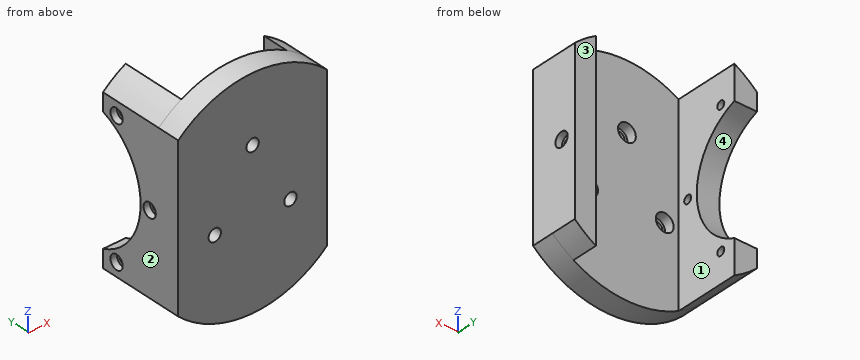
```python
from build123d import *

# Parameters (mm, degrees)
SKETCH8_R            = 1.912019499
BOSS_EXTRUDE7_DEPTH  = 7
SKETCH9_R            = 2.75
CUT_EXTRUDE4_DEPTH   = 3
BOSS_EXTRUDE9_DEPTH  = 20
SKETCH13_R           = 20.5
CUT_EXTRUDE7_DEPTH   = 19.5
SKETCH14_R           = 1.25
CUT_EXTRUDE8_DEPTH   = 19.5
SKETCH15_R           = 2.2
CUT_EXTRUDE9_DEPTH   = 2
BOSS_EXTRUDE10_DEPTH = 8
SKETCH17_R           = 1.25
CUT_EXTRUDE10_DEPTH  = 7.5
CUT_EXTRUDE11_START  = -2
SKETCH18_R           = 2.2
CUT_EXTRUDE11_DEPTH  = 2


with BuildPart() as part:
    # Sketch8 → Boss-Extrude7 (new body)
    with BuildSketch(Plane(origin=(0, 0, 0), x_dir=(1, 0, 0), z_dir=(0, 1, 0))):
        with BuildLine():
            Line((-23, 24.739070187), (-23, -24.739070187))
            ThreePointArc((-23, -24.739070187), (0, -33.779011142), (23, -24.739070187))
            Line((23, -24.739070187), (23, 24.739070187))
            ThreePointArc((23, 24.739070187), (0, 33.779011142), (-23, 24.739070187))
        make_face()
        with Locations(Location((11.691342951, 6.75, 0), (0, 0, 270))):
            Circle(SKETCH8_R, mode=Mode.SUBTRACT)
        with Locations(Location((0, -13.5, 0), (0, 0, 270))):
            Circle(SKETCH8_R, mode=Mode.SUBTRACT)
        with Locations(Location((-11.691342951, 6.75, 0), (0, 0, 270))):
            Circle(SKETCH8_R, mode=Mode.SUBTRACT)
    extrude(amount=BOSS_EXTRUDE7_DEPTH)

    # Sketch9 → Cut-Extrude4 (cut)
    with BuildSketch(Plane(origin=(0, 7, 0), x_dir=(1, 0, 0), z_dir=(0, 1, 0))):
        with Locations(Location((-11.691342951, 6.75, 0), (0, 0, 270))):
            Circle(SKETCH9_R)
        with Locations(Location((11.691342951, 6.75, 0), (0, 0, 270))):
            Circle(SKETCH9_R)
        with Locations(Location((0, -13.5, 0), (0, 0, 270))):
            Circle(SKETCH9_R)
    extrude(amount=-CUT_EXTRUDE4_DEPTH, mode=Mode.SUBTRACT)

    # Sketch12 → Boss-Extrude9 (add)
    with BuildSketch(Plane(origin=(0, 7, 0), x_dir=(1, 0, 0), z_dir=(0, 1, 0))):
        with BuildLine():
            Line((-16, 29.749312491), (-16, -29.749312491))
            ThreePointArc((-16, -29.749312491), (-19.660255135, -27.468089881), (-23, -24.739070187))
            Line((-23, -24.739070187), (-23, 24.739070187))
            ThreePointArc((-23, 24.739070187), (-19.660255135, 27.468089881), (-16, 29.749312491))
        make_face()
    extrude(amount=BOSS_EXTRUDE9_DEPTH)

    # Sketch13 → Cut-Extrude7 (cut)
    with BuildSketch(Plane(origin=(-16, 0, 0), x_dir=(0, 0, -1), z_dir=(1, 0, 0))):
        with Locations((0, 34)):
            Circle(SKETCH13_R)
    extrude(amount=-CUT_EXTRUDE7_DEPTH, mode=Mode.SUBTRACT)

    # Sketch14 → Cut-Extrude8 (cut)
    with BuildSketch(Plane(origin=(-16, 0, 0), x_dir=(0, 0, -1), z_dir=(1, 0, 0))):
        with Locations((0, 10.25)):
            Circle(SKETCH14_R)
        with Locations((-20.56810334, 22.125)):
            Circle(SKETCH14_R)
        with Locations((20.56810334, 22.125)):
            Circle(SKETCH14_R)
    extrude(amount=-CUT_EXTRUDE8_DEPTH, mode=Mode.SUBTRACT)

    # Sketch15 → Cut-Extrude9 (cut)
    with BuildSketch(Plane.ZY.offset(23)):
        with Locations((0, 10.25)):
            Circle(SKETCH15_R)
        with Locations((-20.56810334, 22.125)):
            Circle(SKETCH15_R)
        with Locations((20.56810334, 22.125)):
            Circle(SKETCH15_R)
    extrude(amount=-CUT_EXTRUDE9_DEPTH, mode=Mode.SUBTRACT)

    # Sketch16 → Boss-Extrude10 (add)
    with BuildSketch(Plane(origin=(0, 7, 0), x_dir=(1, 0, 0), z_dir=(0, 1, 0))):
        with BuildLine():
            Line((16.5, 29.474931615), (16.5, -29.474931615))
            ThreePointArc((16.5, -29.474931615), (19.891445294, -27.301135468), (23, -24.739070187))
            Line((23, -24.739070187), (23, 24.739070187))
            ThreePointArc((23, 24.739070187), (19.891445294, 27.301135468), (16.5, 29.474931615))
        make_face()
    extrude(amount=BOSS_EXTRUDE10_DEPTH)

    # Sketch17 → Cut-Extrude10 (cut)
    with BuildSketch(Plane(origin=(23, 0, 0), x_dir=(0, 0, -1), z_dir=(1, 0, 0))):
        with Locations((0, 10.25)):
            Circle(SKETCH17_R)
    extrude(amount=-CUT_EXTRUDE10_DEPTH, mode=Mode.SUBTRACT)

    # Sketch18 → Cut-Extrude11 (cut)
    with BuildSketch(Plane(origin=(23, 0, 0), x_dir=(0, 0, -1), z_dir=(1, 0, 0)).offset(CUT_EXTRUDE11_START)):
        with Locations(Location((0, 10.25, 0), (0, 0, 180))):
            Circle(SKETCH18_R)
    extrude(amount=CUT_EXTRUDE11_DEPTH, mode=Mode.SUBTRACT)


solid = part.part
```
Build history of the part. All positions in model axes, mm. Face numbers are marked on the shaded views. A direction names the side the tool comes from. Coordinates: 2 decimals unless noted, no trailing zeros. Order: outer loops, then holes, each group sorted by start corner. A loop starts at its lowest first (then second) coordinate and runs counter-clockwise, first axis right, second up. Notation, with made-up numbers: (-22, -35.5) -> (0, -35.5) arc R19 ccw to (0, -26.5) -> close; hole circle Ø8 at (85.5, 27). An arc over 180 degrees is marked (long way). Answer in a Markdown table with one row per item. Add a question column.
Q1. Which spindle directions (+Z, -Z, +X, -X, +Y, -Y) get a long thin tool onto all of the face, cutting with end or side? Do the marked faces 1 and 2. Say none if no direction does.
Q2. Band-saw the part on C-C, the plane z = -6.75. List the corners of the cut face in (x, y).
Q3. Band-saw the part on B-B, the plane y = 10.25. List the corners of the cut face in (x, z).
Q4. Band-saw the part on D-D, the plane z = 13.5. List the corners of the cut face in (x, y).
Q5. Drop flat-ended pins along their axis: pin 1 (1.5 mm diameter, centred on x = 10, z = -19, fed in from -Y); pin 2 (1.3 mm diameter, centred on y = 11, z = 0.5, fed in from +X); pin 3 (5 mm diameter, centred on y = 19.5, z = -3.5, fed in from +X); pin 4 (3 mm diameter, centred on x = 1.5, z = 14.5, fed in from +Y). Give the stop position or say it passes through.
Q6. Wall check: line 1 along X through (y, z) = (3.15, -6.75); line 2 along X through (y, z) = (10, -9.5); line 3 along Z through (x, y) = (-20.5, 22). Give the ranges that are in metal, low to high. Write a range as [from, to].
Q7. Mould opens along Z. For the marked faces 3 and 4 say: +Z half, -Z half, draft (parallel to the pull), parting line (faces both ways), or undercut.
Q8. Band-saw the part on A-A, the plane x = 0. List the corners of the cut face in (y, z), then the cut area to 3 significant figures.
Answers follow:
| question | item | result |
|---|---|---|
| 1 | face 1 | +Z, -Z, +Y |
| 1 | face 2 | +Z, -Z, -X, +Y, -Y |
| 2 | outline | (-23, 0) -> (-13.6, 0) -> (-13.6, 4) -> (-14.44, 4) -> (-14.44, 7) -> (-16, 7) -> (-16, 14.64) -> (-23, 14.64) -> close; (-9.78, 0) -> (9.78, 0) -> (9.78, 4) -> (8.94, 4) -> (8.94, 7) -> (-8.94, 7) -> (-8.94, 4) -> (-9.78, 4) -> close; (13.6, 0) -> (23, 0) -> (23, 15) -> (16.5, 15) -> (16.5, 7) -> (14.44, 7) -> (14.44, 4) -> (13.6, 4) -> close |
| 3 | outline | (-23, -24.74) arc R33.78 ccw to (-16, -29.75) -> (-16, -1.25) -> (-21, -1.25) -> (-21, -2.2) -> (-23, -2.2) -> close; (-23, 2.2) -> (-21, 2.2) -> (-21, 1.25) -> (-16, 1.25) -> (-16, 29.75) arc R33.78 ccw to (-23, 24.74) -> close; (16.5, -29.47) arc R33.78 ccw to (23, -24.74) -> (23, -2.2) -> (21, -2.2) -> (21, -1.25) -> (16.5, -1.25) -> close; (16.5, 1.25) -> (21, 1.25) -> (21, 2.2) -> (23, 2.2) -> (23, 24.74) arc R33.78 ccw to (16.5, 29.47) -> close |
| 4 | outline | (-23, 0) -> (-1.91, 0) -> (-1.91, 4) -> (-2.75, 4) -> (-2.75, 7) -> (-16, 7) -> (-16, 18.57) -> (-23, 18.57) -> close; (1.91, 0) -> (23, 0) -> (23, 15) -> (16.5, 15) -> (16.5, 7) -> (2.75, 7) -> (2.75, 4) -> (1.91, 4) -> close |
| 5 | pin 1 | y = 0 |
| 5 | pin 2 | x = 21 |
| 5 | pin 3 | through |
| 5 | pin 4 | y = 7 |
| 6 | line 1 | [-23, -13.6], [-9.78, 9.78], [13.6, 23] |
| 6 | line 2 | [-23, -16], [16.5, 23] |
| 6 | line 3 | [-26.85, -21.81], [-19.32, -16.62], [16.62, 19.32], [21.81, 26.85] |
| 7 | face 3 | draft |
| 7 | face 4 | undercut |
| 8 | outline | (0, -33.78) -> (7, -33.78) -> (7, 10.75) -> (4, 10.75) -> (4, 11.59) -> (0, 11.59) -> close; (0, 15.41) -> (4, 15.41) -> (4, 16.25) -> (7, 16.25) -> (7, 33.78) -> (0, 33.78) -> close |
| 8 | area | 441 mm^2 |
